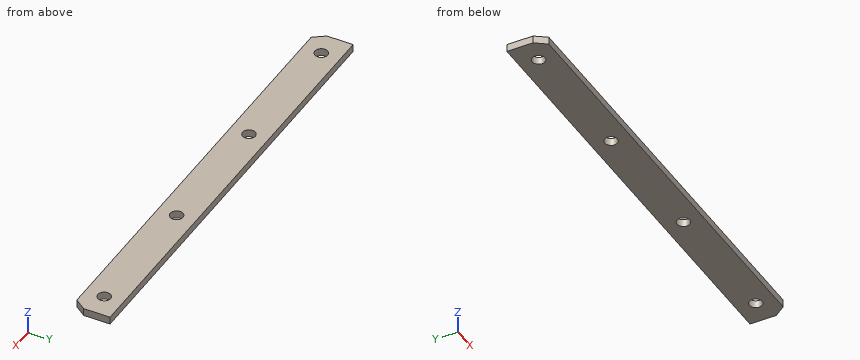
from build123d import *

# Parameters (mm, degrees)
SKETCH1_W               = 270
SKETCH1_H               = 10
BOSS_EXTRUDE1_DEPTH     = 2
CHAMFER1_SIZE           = 2
M3_CLEARANCE_HOLE1_D    = 3.4
LPATTERN1_COUNT         = 8
LPATTERN1_PITCH         = 35.714285714
CUT_EXTRUDE_THIN1_DEPTH = 10


with BuildPart() as part:
    # Sketch1 → Boss-Extrude1 (new body)
    with BuildSketch(Plane.XY):
        Rectangle(SKETCH1_W, SKETCH1_H)
    extrude(amount=BOSS_EXTRUDE1_DEPTH)

    # Chamfer1
    chamfer1_edges = [part.edges().sort_by_distance(p)[0] for p in [
        (135, -5, 1),
        (-135, -5, 1),
    ]]
    chamfer(chamfer1_edges, length=CHAMFER1_SIZE)

    # M3 Clearance Hole1 (through all)
    with Locations(Plane.XY.offset(2)):
        with Locations((125, 0)):
            m3_clearance_hole1 = Hole(M3_CLEARANCE_HOLE1_D / 2)

    # LPattern1: M3 Clearance Hole1 ×8
    with Locations(*[(-i * LPATTERN1_PITCH, 0, 0) for i in range(1, LPATTERN1_COUNT)]):
        add(m3_clearance_hole1, mode=Mode.SUBTRACT)

    # Sketch4 → Cut-Extrude-Thin1 (cut)
    with BuildSketch(Plane(origin=(0, 0, 0), x_dir=(-1, 0, 0), z_dir=(0, 0, -1))):
        Polygon((160, 105), (-160, 105), (-160, -34.491969623), (-108.772917365, -105), (108.772917365, -105), (160, -34.491969623), align=None)
        Polygon((60, 5), (-60, 5), (-60, -2), (-57.820372416, -5), (57.820372416, -5), (60, -2), align=None, mode=Mode.SUBTRACT)
    extrude(amount=-CUT_EXTRUDE_THIN1_DEPTH, mode=Mode.SUBTRACT)


solid = part.part
Here's how the part is built. I have some questions about the finished solid (model axes, mm). Give positions to 0.01 mm unless a question says otherwise; leave off trailing zeros. Order: outer loops, then holes, each group sorted by start corner. A loop starts at its lowest first (then second) coordinate and runs counter-clockwise, first axis right, second up. Notation, with made-up numbers: (-27.75, -12) -> (27.25, -12) arc R10 cw to (27.25, -2) -> close; hole circle Ø10 at (78.5, 3.25). An arc over 180 degrees is marked (long way). One line per item, written item: value. Start each with the question number.
1. Imagine slicing it at A-A, the plane z = 1.05. List the corners of the cut face in (x, y) for me.
2. Imagine slicing it at B-B, the plane y = 0. List the corners of the cut face in (x, z) for me.
3. Imagine slicing it at C-C, the plane x = -18.5. List the corners of the cut face in (y, z) for me.
4. Will this pin go through, and if not, where does the flat tip stop? pin 1 Ø2 at (x, y) = (-17.86, 0) entering from +Z.
5. I need wall thicknesses on probe 1 along X at (y, z) = (-0.75, 0.9); probe 2 along X at (y, z) = (1, 0.65); probe 3 along Y at (x, z) = (-53, 1.9). Which ranges of each line are inside material? Lowest first, please. Write a range as from..to.
Values follow:
1. outline: (-60, -2) -> (-57.82, -5) -> (57.82, -5) -> (60, -2) -> (60, 5) -> (-60, 5) -> close; hole circle Ø3.4 at (-53.57, 0); hole circle Ø3.4 at (-17.86, 0); hole circle Ø3.4 at (17.86, 0); hole circle Ø3.4 at (53.57, 0)
2. outline: (-60, 0) -> (-55.27, 0) -> (-55.27, 2) -> (-60, 2) -> close; (-51.87, 0) -> (-19.56, 0) -> (-19.56, 2) -> (-51.87, 2) -> close; (-16.16, 0) -> (16.16, 0) -> (16.16, 2) -> (-16.16, 2) -> close; (19.56, 0) -> (51.87, 0) -> (51.87, 2) -> (19.56, 2) -> close; (55.27, 0) -> (60, 0) -> (60, 2) -> (55.27, 2) -> close
3. outline: (-5, 0) -> (-1.57, 0) -> (-1.57, 2) -> (-5, 2) -> close; (1.57, 0) -> (5, 0) -> (5, 2) -> (1.57, 2) -> close
4. pin 1: passes through
5. probe 1: x = -60..-55.1, -52.05..-19.38, -16.33..16.33, 19.38..52.05, 55.1..60
5. probe 2: x = -60..-54.95, -52.2..-19.23, -16.48..16.48, 19.23..52.2, 54.95..60
5. probe 3: y = -5..-1.6, 1.6..5
